For this review, take the finished solid that the model builds, in its own axes (mm). Coordinates: 2 decimals unless noted, no trailing zeros. Loops run counter-clockwise (first coordinate to the right, second up) from the corner with the lowest first, then second, coordinate; pieces in that order, holes last. Notation, with made-up numbers: (74.25, 0.5) -> (86.25, 0.5) arc R13 cw to (86.25, 22.5) -> close; hole circle Ø8 at (68.25, -8). An arc over 180 degrees is marked (long way). Answer in a Markdown table with one row per item.
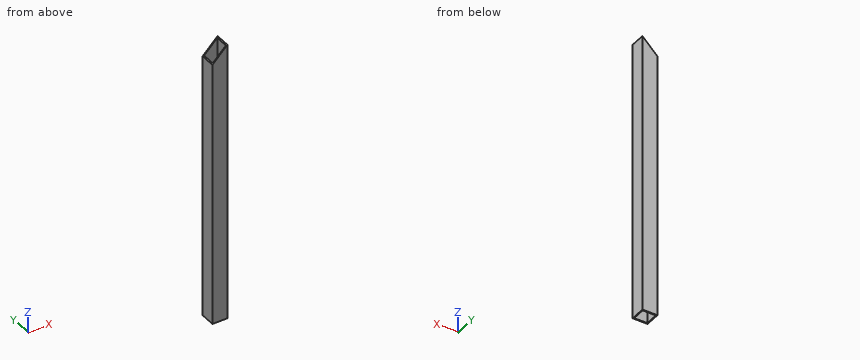
Autodesk Inventor part; units mm, degrees
ref_plane "YZ Plane" through (0, 0, 0) normal (1, 0, 0) x (0, 1, 0)
ref_plane "XZ Plane" through (0, 0, 0) normal (0, 1, 0) x (-1, 0, 0)
ref_plane "XY Plane" through (0, 0, 0) normal (0, 0, 1) x (1, 0, 0)
sketch "Sketch1" plane through (0, 0, 0) normal (0, 0, 1) x (1, 0, 0)
  line L0 (0, 0) -> (25.4, 0)
  line L1 (25.4, 0) -> (25.4, 25.4)
  line L2 (25.4, 25.4) -> (0, 25.4)
  line L3 (0, 25.4) -> (0, 0)
  line L4 (1.5875, 1.5875) -> (23.8125, 1.5875)
  line L5 (23.8125, 1.5875) -> (23.8125, 23.8125)
  line L6 (23.8125, 23.8125) -> (1.5875, 23.8125)
  line L7 (1.5875, 23.8125) -> (1.5875, 1.5875)
  dimension "d0" = 25.4
  dimension "d1" = 25.4
  dimension "d2" = 1.5875
extrude "Extrusion1" add sketch "Sketch1" along normal blind 478.8916
sketch "Sketch2" plane through (0, 25.4, 0) normal (0, 1, 0) x (1, 0, 0)
  line L0 (0, -478.8916) -> (25.4, -478.8916)
  line L1 (25.4, -478.8916) -> (0, -453.4916)
  line L2 (0, -453.4916) -> (0, -478.8916)
  line L3 (0, -478.8916) -> (25.4, -478.8916)
  point P0 (0, 0)
  dimension "d5" = 25.4
extrude "Extrusion2" cut sketch "Sketch2" against normal blind 25.4
properties part number "SUP_007_ConnectorBar" material "Aluminum 6061"
Item 1: For L1, parallel to X at y = 12, z = 322; L2, parallel to X at y = 23.5, z = 456.5, list the stretches that pass through material, from the lowest coordinate up.
Worked answers:
| item | result |
|---|---|
| L1 | 0 to 1.59, 23.81 to 25.4 |
| L2 | 23.81 to 25.4 |
Item 2: Take a section at A-A, the plane y = 17. State the section outline as (x, z) points, and give its area (3 significant figures).
Worked answers:
| item | result |
|---|---|
| outline | (0, 0) -> (1.59, 0) -> (1.59, 455.08) -> (0, 453.49) -> close; (23.81, 0) -> (25.4, 0) -> (25.4, 478.89) -> (23.81, 477.3) -> close |
| area | 1,480 mm² |
Item 3: Take a section at B-B, the plane x = 12.5. State the section outline as (y, z) points.
Worked answers:
| item | result |
|---|---|
| outline | (0, 0) -> (1.59, 0) -> (1.59, 465.99) -> (0, 465.99) -> close; (23.81, 0) -> (25.4, 0) -> (25.4, 465.99) -> (23.81, 465.99) -> close |
Item 4: Insertion check: pin 1 (5 mm diameter, centred on x = 10, y = 4.5, fed in from -Z). The pin has a flat end and moves straight along its axis. Give the tip position at first contact, or say it passes through.
Worked answers:
| item | result |
|---|---|
| pin 1 | through |
Item 5: Take a section at C-C, the plane z = 54. State the section outline as (x, y) points, and give its area (3 significant figures).
Worked answers:
| item | result |
|---|---|
| outline | (0, 0) -> (25.4, 0) -> (25.4, 25.4) -> (0, 25.4) -> close; hole (1.59, 1.59) -> (23.81, 1.59) -> (23.81, 23.81) -> (1.59, 23.81) -> close |
| area | 151 mm² |
